Print and shaded views of the part. All mm, measured from the part's lowest x, y and z. A direction names the side the tool comes from. Give positions to 0.01 mm unless a question says otherwise; leave off trailing zeros. Loops run counter-clockwise (first coordinate to the right, second up) from the corner with the lowest first, then second, coordinate; pieces in that order, holes last. Notation, with made-up numbers: M -34.75,-26 L 14.25,-26 A21 ccw 14.25,-19 Z; hole C 55.25,83.25 d6. An arc over 180 degrees is marked long. Answer as CSV lines item,"result".
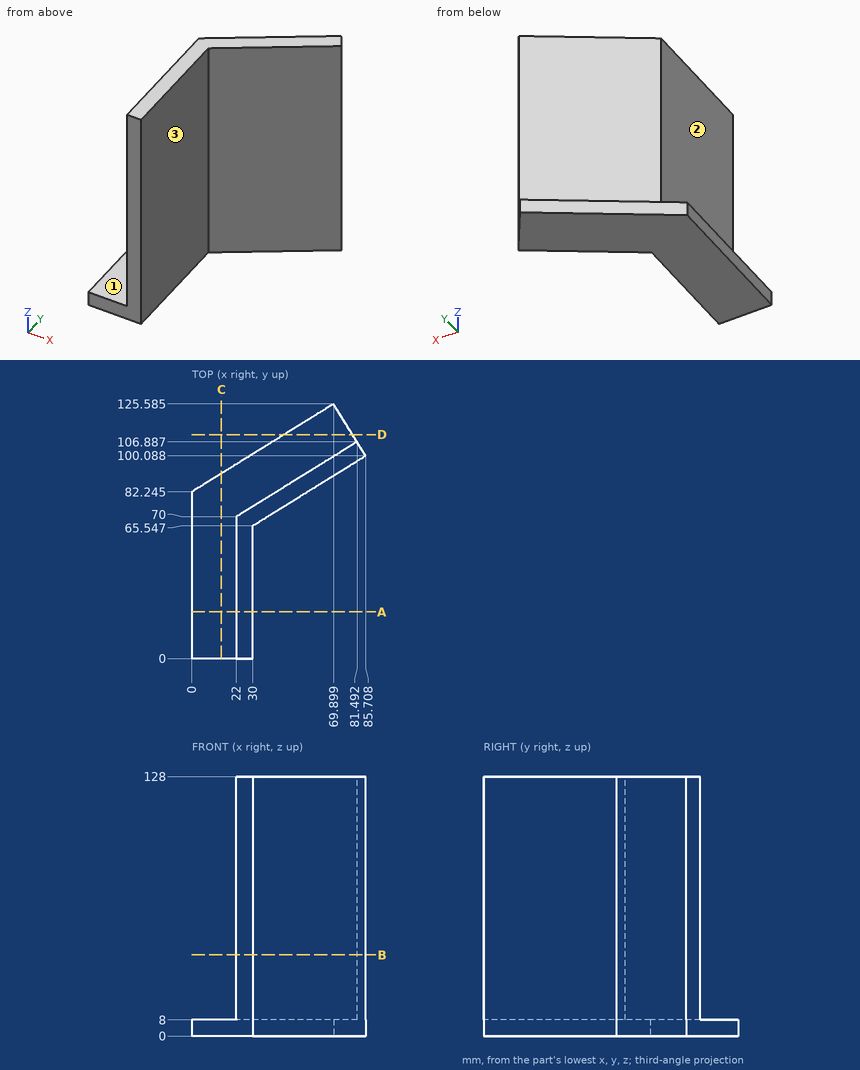
Q1. Cut at D-D (y = 110.5). Write the cut outline in (x, z).
Solution:
outline,"M 45.57,0 L 79.25,0 L 79.25,8 L 45.57,8 Z"
Q2. Cut at A-A (y = 23). Write the cut outline in (x, z).
Solution:
outline,"M 0,0 L 30,0 L 30,128 L 22,128 L 22,8 L 0,8 Z"
Q3. Which spindle directions (+Z, -Z, +X, -X, +Y, -Y) get a long thin tool onto all of the face, cutting with end or side? Do the marked faces 1, 2 and 3. Say none if no direction does.
Solution:
face 1,"+Z, -X, +Y"
face 2,"+Z, -X, +Y, -Y"
face 3,"+Z, -Z, +X, -Y"
Q4. Wall check: line 1 (Z direction, x = 8.5, y = 43); line 2 (X direction, y = 13, z = 34.5); line 3 (X direction, y = 45.5, z = 7). Give the ranges that are in metal, low to high. Write a range as [from, to].
Solution:
line 1,"z = [0, 8]"
line 2,"x = [22, 30]"
line 3,"x = [0, 30]"
Q5. Pin check, flat tips, straight feed: P1, Ø3, axis at x = 72.5, z = 45, coming from the +Y side; P2, Ø19.5, axis at y = 24.5, z = 70, coming from the +X side; P3, Ø3, axis at y = 43, z = 46, coming from the -X side. Stop position of each tip, or through.
Solution:
P1,"stops at y = 102.24"
P2,"stops at x = 30"
P3,"stops at x = 22"
Q6. Cut at C-C (x = 14.5). Write the cut outline in (y, z) (1 decimal), and give its area (3 significant figures).
Solution:
outline,"M 0,0 L 91.2,0 L 91.2,8 L 0,8 Z"
area,"730 mm²"
Q7. Cut at B-B (z = 40). Write the cut outline in (x, y).
Solution:
outline,"M 22,0 L 30,0 L 30,65.55 L 85.71,100.09 L 81.49,106.89 L 22,70 Z"
